from build123d import *

# Parameters (mm, degrees)
BOSS_EXTRUDE1_DEPTH = 114
SKETCH3_W           = 82.5
SKETCH3_H           = 94
CUT_EXTRUDE1_DEPTH  = 3
CUT_EXTRUDE2_DEPTH  = 17
SKETCH5_R           = 19
BOSS_EXTRUDE2_DEPTH = 3
SKETCH6_R           = 47.5
SKETCH6_R_2         = 31
BOSS_EXTRUDE4_DEPTH = 61
SKETCH8_W           = 3
SKETCH8_H           = 35.544994967
SKETCH9_R           = 1.5
CUT_EXTRUDE3_DEPTH  = 22


with BuildPart() as part:
    # Sketch2 → Boss-Extrude1 (new body)
    with BuildSketch(Plane.XY):
        Polygon((-102, 0), (-97, 16), (97, 16), (102, 0), align=None)
    extrude(amount=-BOSS_EXTRUDE1_DEPTH)

    # Sketch3 → Cut-Extrude1 (cut)
    with BuildSketch(Plane.XZ):
        with Locations((-50.75, -57)):
            Rectangle(SKETCH3_W, SKETCH3_H)
        with Locations((50.75, -57)):
            Rectangle(SKETCH3_W, SKETCH3_H)
    extrude(amount=-CUT_EXTRUDE1_DEPTH, mode=Mode.SUBTRACT)

    # Sketch4 → Cut-Extrude2 (cut, through all)
    with BuildSketch(Plane(origin=(0, 16, 0), x_dir=(1, 0, 0), z_dir=(0, 1, 0))):
        with BuildLine():
            Line((-76, 77), (-70, 77))
            ThreePointArc((-70, 77), (-62, 85), (-70, 93))
            Line((-70, 93), (-76, 93))
            ThreePointArc((-76, 93), (-84, 85), (-76, 77))
        make_face()
        with BuildLine():
            ThreePointArc((70, 77), (62, 85), (70, 93))
            Line((70, 93), (76, 93))
            ThreePointArc((76, 93), (84, 85), (76, 77))
            Line((76, 77), (70, 77))
        make_face()
        with BuildLine():
            ThreePointArc((-70, 37), (-62, 29), (-70, 21))
            Line((-70, 21), (-76, 21))
            ThreePointArc((-76, 21), (-84, 29), (-76, 37))
            Line((-76, 37), (-70, 37))
        make_face()
        with BuildLine():
            Line((76, 37), (70, 37))
            ThreePointArc((70, 37), (62, 29), (70, 21))
            Line((70, 21), (76, 21))
            ThreePointArc((76, 21), (84, 29), (76, 37))
        make_face()
    extrude(amount=-CUT_EXTRUDE2_DEPTH, mode=Mode.SUBTRACT)

    # Sketch5 → Boss-Extrude2 (add)
    with BuildSketch(Plane(origin=(0, 16, 0), x_dir=(1, 0, 0), z_dir=(0, 1, 0))):
        with Locations(Location((-73, 85, 0), (0, 0, 180))):  # turned: the seam where the file's is
            Circle(SKETCH5_R)
        with BuildLine():
            ThreePointArc((-70, 93), (-62, 85), (-70, 77))
            Line((-70, 77), (-76, 77))
            ThreePointArc((-76, 77), (-84, 85), (-76, 93))
            Line((-76, 93), (-70, 93))
        make_face(mode=Mode.SUBTRACT)
        with Locations(Location((73, 85, 0), (0, 0, 180))):  # turned: the seam where the file's is
            Circle(SKETCH5_R)
        with BuildLine():
            ThreePointArc((76, 93), (84, 85), (76, 77))
            Line((76, 77), (70, 77))
            ThreePointArc((70, 77), (62, 85), (70, 93))
            Line((70, 93), (76, 93))
        make_face(mode=Mode.SUBTRACT)
        with Locations(Location((73, 29, 0), (0, 0, 180))):  # turned: the seam where the file's is
            Circle(SKETCH5_R)
        with BuildLine():
            ThreePointArc((70, 21), (62, 29), (70, 37))
            Line((70, 37), (76, 37))
            ThreePointArc((76, 37), (84, 29), (76, 21))
            Line((76, 21), (70, 21))
        make_face(mode=Mode.SUBTRACT)
        with Locations(Location((-73, 29, 0), (0, 0, 180))):  # turned: the seam where the file's is
            Circle(SKETCH5_R)
        with BuildLine():
            ThreePointArc((-76, 21), (-84, 29), (-76, 37))
            Line((-76, 37), (-70, 37))
            ThreePointArc((-70, 37), (-62, 29), (-70, 21))
            Line((-70, 21), (-76, 21))
        make_face(mode=Mode.SUBTRACT)
    extrude(amount=BOSS_EXTRUDE2_DEPTH)

    # Sketch6 → Boss-Extrude4 (add)
    with BuildSketch(Plane(origin=(0, 16, 0), x_dir=(1, 0, 0), z_dir=(0, 1, 0))):
        with Locations(Location((0, 57, 0), (0, 0, 180))):  # turned: the seam where the file's is
            Circle(SKETCH6_R)
        with Locations(Location((0, 57, 0), (0, 0, 180))):  # turned: the seam where the file's is
            Circle(SKETCH6_R_2, mode=Mode.SUBTRACT)
    extrude(amount=BOSS_EXTRUDE4_DEPTH)

    # Sketch8 → Cut-Revolve1 (revolve, cut)
    with BuildSketch(Plane.XY.offset(-57)):
        with Locations((-31, 48.227502517)):
            Rectangle(SKETCH8_W, SKETCH8_H)
    revolve(axis=Axis((0, 107.106199385, -57), (0, -1, 0)), mode=Mode.SUBTRACT)

    # Sketch9 → Cut-Extrude3 (cut)
    with BuildSketch(Plane(origin=(0, 16, 0), x_dir=(1, 0, 0), z_dir=(0, 1, 0))):
        with Locations(Location((-22, 57, 0), (0, 0, 180))):  # turned: the seam where the file's is
            Circle(SKETCH9_R)
    extrude(amount=-CUT_EXTRUDE3_DEPTH, mode=Mode.SUBTRACT)


solid = part.part
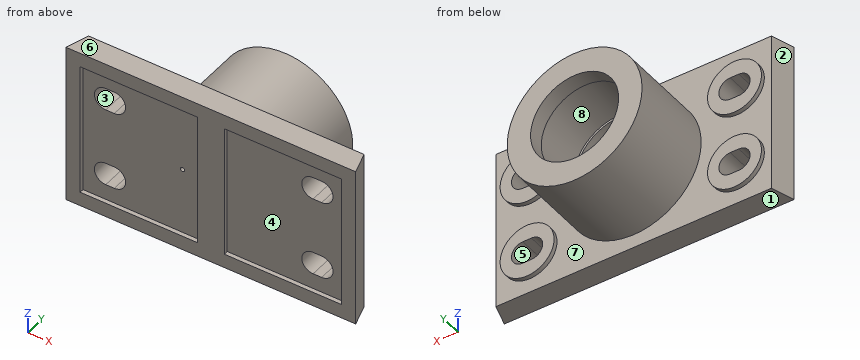
Work out the finished part from the listing and answer in its coordinate system (mm). Face numbers are marked on the shaded views. A direction names the side the tool comes from. Give positions to 0.01 mm unless a question says otherwise; leave off trailing zeros. Loops run counter-clockwise (first coordinate to the right, second up) from the corner with the lowest first, then second, coordinate; pieces in that order, holes last. Notation, with made-up numbers: M 47.5,-4 L 97.5,-4 A16 cw 97.5,9 Z; hole C 27.5,48.25 d5. An arc over 180 degrees is marked long. Use CSV: the item, a comma, the result in double quotes.
1) Find section A-A on x = 0. Write down the section's boundary in (y, z) (3 decimals).
Answer:
outline,"M 0,-114 L 16,-114 L 16,-104.5 L 77,-104.5 L 77,-88 L 66,-88 L 66,-89.5 L 30.455,-89.5 L 30.455,-88 L 16,-88 L 16,-26 L 30.455,-26 L 30.455,-24.5 L 66,-24.5 L 66,-26 L 77,-26 L 77,-9.5 L 16,-9.5 L 16,0 L 0,0 Z"
2) Which of the six approach directions +Z, -Z, +X, -X, +Y, -Y give full straight-line access (tool end or side, diameter ignored) to the marked faces 4, 5, 6, 7 and 8?
Answer:
face 4,"-Y"
face 5,"+Y, -Y"
face 6,"+Z, +X, -X, +Y, -Y"
face 7,"+Y"
face 8,"none"
3) Find section C-C on x = 67.5. Write down the section's boundary in (y, z).
Answer:
outline,"M 0,-114 L 16,-114 L 16,-103.19 L 19,-103.19 L 19,-92.6 L 3,-92.6 L 3,-104 L 0,-104 Z; M 0,-10 L 3,-10 L 3,-21.4 L 19,-21.4 L 19,-10.81 L 16,-10.81 L 16,0 L 0,0 Z; M 3,-77.4 L 19,-77.4 L 19,-66.81 L 16,-66.81 L 16,-47.19 L 19,-47.19 L 19,-36.6 L 3,-36.6 Z"
4) Find section B-B on y = 10. Write down the section's boundary in (x, z) (3 decimals).
Answer:
outline,"M -98.875,-114 L 98.875,-114 L 98.875,0 L -98.875,0 Z; hole M -76,-93 L -70,-93 A8 ccw -70,-77 L -76,-77 A8 ccw Z; hole M -76,-37 L -70,-37 A8 ccw -70,-21 L -76,-21 A8 ccw Z; hole C -22,-57 d3; hole M 70,-93 L 76,-93 A8 ccw 76,-77 L 70,-77 A8 ccw Z; hole M 70,-37 L 76,-37 A8 ccw 76,-21 L 70,-21 A8 ccw Z"
5) Find section D-D on y = 64. Write down the section's boundary in (x, z), plus the area to 3 significant figures.
Answer:
outline,"C 0,-57 d95; hole C 0,-57 d65"
area,"3,770 mm^2"
6) Given P1, Ø4, axis at x = 4.5, z = -52.5, coming from the +Y side; P2, Ø1.5, axis at x = -42.5, y = 23, coming from the -Z side; P3, Ø2, axis at x = -75, z = -46, coming from the -Y side, each flat-ended and moving along its own axis, determine where each tip first touches the part or whether it passes through.
Answer:
P1,"y = 16"
P2,"z = -79.65"
P3,"y = 3"
7) Determine the mould class of the marked faces 1, 2 and 3 for opening direction X: released by +X, released by -X, zero draft, split by the parting line, or undercut.
Answer:
face 1,"zero draft"
face 2,"released by -X"
face 3,"undercut"
8) Consider L1, parallel to Z at x = 0, y = 22.25; L2, parallel to Z at x = 0, y = 49; L3, parallel to X at y = 11.5, z = -82.5. Determine where each line is inside the solid, lowest interval first.
Answer:
L1,"-104.5 to -88, -26 to -9.5"
L2,"-104.5 to -89.5, -24.5 to -9.5"
L3,"-98.41 to -83.6, -62.4 to 62.4, 83.6 to 98.41"
